Can you work these out from the model? Positions are in its coordinate system, mm. Give positions to 0.01 mm unless a question says otherwise; leave off trailing zeros. Order: outer loops, then holes, each group sorted by start corner. A loop starts at its lowest first (then second) coordinate and runs counter-clockwise, first axis right, second up. Notation, with made-up numbers: M -13.75,77 L 39.25,77 A17 cw 39.25,88 Z; hole C 22.5,6.25 d8. An arc over 180 degrees is marked long. One line per question, with ' | ' between items. Start each with the question number.
1) Please list where these lines run through material, in increasing order: line 1 along X through (y, z) = (0.25, -0.5); line 2 along X through (y, z) = (1, -0.05); line 3 along Y through (x, z) = (-44, 0.15). Write a range as [from, to].
2) If we section it at B-B, the plane x = 6.5: Please give me the cut outline in (y, z).
3) If we section it at A-A, the plane y = 0: Please give me the cut outline in (x, z), plus the area to 4 significant figures.
4) If we section it at C-C, the plane z = -0.4: Please give me the cut outline in (x, y).
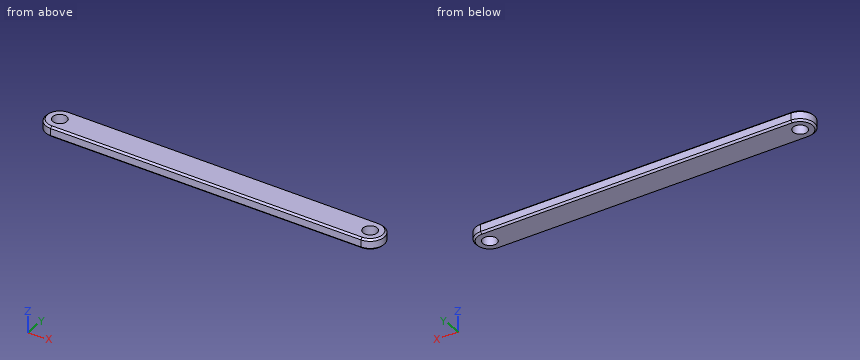
```python
from build123d import *

# Parameters (mm, degrees)
SKETCH1_R           = 2
BOSS_EXTRUDE1_DEPTH = 1.5
CHAMFER1_SIZE       = 0.5


with BuildPart() as part:
    # Sketch1 → Boss-Extrude1 (new body, symmetric)
    with BuildSketch(Plane.XY):
        with BuildLine():
            Line((-44, 4), (44, 4))
            ThreePointArc((44, 4), (48, 0), (44, -4))
            Line((44, -4), (-44, -4))
            ThreePointArc((-44, -4), (-48, 0), (-44, 4))
        make_face()
        with Locations((-44, 0)):
            Circle(SKETCH1_R, mode=Mode.SUBTRACT)
        with Locations((44, 0)):
            Circle(SKETCH1_R, mode=Mode.SUBTRACT)
    extrude(amount=BOSS_EXTRUDE1_DEPTH, both=True)

    # Chamfer1
    chamfer1_edges = [part.edges().sort_by_distance(p)[0] for p in [
        (48, 0, 1.5),
        (0, 4, 1.5),
        (-48, 0, 1.5),
        (0, 4, -1.5),
        (48, 0, -1.5),
        (0, -4, -1.5),
        (-48, 0, -1.5),
        (0, -4, 1.5),
    ]]
    chamfer(chamfer1_edges, length=CHAMFER1_SIZE)


solid = part.part
```
Results found:
1) line 1: x = [-47.99, -45.98], [-42.02, 42.02], [45.98, 47.99] | line 2: x = [-47.87, -45.73], [-42.27, 42.27], [45.73, 47.87] | line 3: y = [-4, -2], [2, 4]
2) outline: M -4,-1 L -3.5,-1.5 L 3.5,-1.5 L 4,-1 L 4,1 L 3.5,1.5 L -3.5,1.5 L -4,1 Z
3) outline: M -48,-1 L -47.5,-1.5 L -46,-1.5 L -46,1.5 L -47.5,1.5 L -48,1 Z; M -42,-1.5 L 42,-1.5 L 42,1.5 L -42,1.5 Z; M 46,-1.5 L 47.5,-1.5 L 48,-1 L 48,1 L 47.5,1.5 L 46,1.5 Z | area: 263.5 mm²
4) outline: M -44,-4 L 44,-4 A4 ccw 44,4 L -44,4 A4 ccw Z; hole C -44,0 d4; hole C 44,0 d4
